Geometry check sheet. Reference: the model listing, model coordinates, mm. A direction names the side the tool comes from. Coordinates: 2 decimals unless noted, no trailing zeros. Write each loop counter-clockwise with the first axis right and the second up, starting at its lowest first coordinate (ties: lowest second). Pieces come first, ordered by that corner, then holes. Notation, with made-up numbers: (74.25, -0.75) -> (130.25, -0.75) arc R19 ccw to (130.25, 15.25) -> close; hole circle Ø2 at (-2, -17). An arc over 180 degrees is marked (long way). Use a Markdown table: item, result.
```python
from build123d import *

# Parameters (mm, degrees)
F1_DEPTH = 6.35
F2_R     = 6.35
F3_DEPTH = 6.35
F4_R     = 7.9375
F4_R_2   = 6.35
F5_DEPTH = 1.5875


with BuildPart() as f1:
    # F0 (on Front) → F1 (new body)
    with BuildSketch(Plane.XZ):
        with BuildLine():
            Line((-1.190625, 4.953), (-1.190625, 6.108039))
            ThreePointArc((-1.190625, 6.108039), (-2.381439, 5.749302), (-3.477137, 5.160935))
            Line((-3.477137, 5.160935), (-2.660401, 4.344199))
            Line((-2.660401, 4.344199), (-4.344199, 2.660401))
            Line((-4.344199, 2.660401), (-5.160935, 3.477137))
            ThreePointArc((-5.160935, 3.477137), (-5.749302, 2.381439), (-6.108039, 1.190625))
            Line((-6.108039, 1.190625), (-4.953, 1.190625))
            Line((-4.953, 1.190625), (-4.953, -1.190625))
            Line((-4.953, -1.190625), (-6.108039, -1.190625))
            ThreePointArc((-6.108039, -1.190625), (-5.749302, -2.381439), (-5.160935, -3.477137))
            Line((-5.160935, -3.477137), (-4.344199, -2.660401))
            Line((-4.344199, -2.660401), (-2.660401, -4.344199))
            Line((-2.660401, -4.344199), (-3.477137, -5.160935))
            ThreePointArc((-3.477137, -5.160935), (-2.381439, -5.749302), (-1.190625, -6.108039))
            Line((-1.190625, -6.108039), (-1.190625, -4.953))
            Line((-1.190625, -4.953), (1.190625, -4.953))
            Line((1.190625, -4.953), (1.190625, -6.108039))
            ThreePointArc((1.190625, -6.108039), (2.381439, -5.749302), (3.477137, -5.160935))
            Line((3.477137, -5.160935), (2.660401, -4.344199))
            Line((2.660401, -4.344199), (4.344199, -2.660401))
            Line((4.344199, -2.660401), (5.160935, -3.477137))
            ThreePointArc((5.160935, -3.477137), (5.749302, -2.381439), (6.108039, -1.190625))
            Line((6.108039, -1.190625), (4.953, -1.190625))
            Line((4.953, -1.190625), (4.953, 1.190625))
            Line((4.953, 1.190625), (6.108039, 1.190625))
            ThreePointArc((6.108039, 1.190625), (5.749302, 2.381439), (5.160935, 3.477137))
            Line((5.160935, 3.477137), (4.344199, 2.660401))
            Line((4.344199, 2.660401), (2.660401, 4.344199))
            Line((2.660401, 4.344199), (3.477137, 5.160935))
            ThreePointArc((3.477137, 5.160935), (2.381439, 5.749302), (1.190625, 6.108039))
            Line((1.190625, 6.108039), (1.190625, 4.953))
            Line((1.190625, 4.953), (-1.190625, 4.953))
        make_face()
    extrude(amount=F1_DEPTH)

    # F2 (on face) → F3 (join)
    with BuildSketch(Plane.XZ.offset(6.35)):
        Circle(F2_R)
        with BuildLine():
            Line((-3.477137, -5.160935), (-2.660401, -4.344199))
            Line((-2.660401, -4.344199), (-4.344199, -2.660401))
            Line((-4.344199, -2.660401), (-5.160935, -3.477137))
            ThreePointArc((-5.160935, -3.477137), (-5.749302, -2.381439), (-6.108039, -1.190625))
            Line((-6.108039, -1.190625), (-4.953, -1.190625))
            Line((-4.953, -1.190625), (-4.953, 1.190625))
            Line((-4.953, 1.190625), (-6.108039, 1.190625))
            ThreePointArc((-6.108039, 1.190625), (-5.749302, 2.381439), (-5.160935, 3.477137))
            Line((-5.160935, 3.477137), (-4.344199, 2.660401))
            Line((-4.344199, 2.660401), (-2.660401, 4.344199))
            Line((-2.660401, 4.344199), (-3.477137, 5.160935))
            ThreePointArc((-3.477137, 5.160935), (-2.381439, 5.749302), (-1.190625, 6.108039))
            Line((-1.190625, 6.108039), (-1.190625, 4.953))
            Line((-1.190625, 4.953), (1.190625, 4.953))
            Line((1.190625, 4.953), (1.190625, 6.108039))
            ThreePointArc((1.190625, 6.108039), (2.381439, 5.749302), (3.477137, 5.160935))
            Line((3.477137, 5.160935), (2.660401, 4.344199))
            Line((2.660401, 4.344199), (4.344199, 2.660401))
            Line((4.344199, 2.660401), (5.160935, 3.477137))
            ThreePointArc((5.160935, 3.477137), (5.749302, 2.381439), (6.108039, 1.190625))
            Line((6.108039, 1.190625), (4.953, 1.190625))
            Line((4.953, 1.190625), (4.953, -1.190625))
            Line((4.953, -1.190625), (6.108039, -1.190625))
            ThreePointArc((6.108039, -1.190625), (5.749302, -2.381439), (5.160935, -3.477137))
            Line((5.160935, -3.477137), (4.344199, -2.660401))
            Line((4.344199, -2.660401), (2.660401, -4.344199))
            Line((2.660401, -4.344199), (3.477137, -5.160935))
            ThreePointArc((3.477137, -5.160935), (2.381439, -5.749302), (1.190625, -6.108039))
            Line((1.190625, -6.108039), (1.190625, -4.953))
            Line((1.190625, -4.953), (-1.190625, -4.953))
            Line((-1.190625, -4.953), (-1.190625, -6.108039))
            ThreePointArc((-1.190625, -6.108039), (-2.381439, -5.749302), (-3.477137, -5.160935))
        make_face(mode=Mode.SUBTRACT)
        with BuildLine():
            Line((-4.344199, -2.660401), (-2.660401, -4.344199))
            Line((-2.660401, -4.344199), (-3.477137, -5.160935))
            ThreePointArc((-3.477137, -5.160935), (-2.381439, -5.749302), (-1.190625, -6.108039))
            Line((-1.190625, -6.108039), (-1.190625, -4.953))
            Line((-1.190625, -4.953), (1.190625, -4.953))
            Line((1.190625, -4.953), (1.190625, -6.108039))
            ThreePointArc((1.190625, -6.108039), (2.381439, -5.749302), (3.477137, -5.160935))
            Line((3.477137, -5.160935), (2.660401, -4.344199))
            Line((2.660401, -4.344199), (4.344199, -2.660401))
            Line((4.344199, -2.660401), (5.160935, -3.477137))
            ThreePointArc((5.160935, -3.477137), (5.749302, -2.381439), (6.108039, -1.190625))
            Line((6.108039, -1.190625), (4.953, -1.190625))
            Line((4.953, -1.190625), (4.953, 1.190625))
            Line((4.953, 1.190625), (6.108039, 1.190625))
            ThreePointArc((6.108039, 1.190625), (5.749302, 2.381439), (5.160935, 3.477137))
            Line((5.160935, 3.477137), (4.344199, 2.660401))
            Line((4.344199, 2.660401), (2.660401, 4.344199))
            Line((2.660401, 4.344199), (3.477137, 5.160935))
            ThreePointArc((3.477137, 5.160935), (2.381439, 5.749302), (1.190625, 6.108039))
            Line((1.190625, 6.108039), (1.190625, 4.953))
            Line((1.190625, 4.953), (-1.190625, 4.953))
            Line((-1.190625, 4.953), (-1.190625, 6.108039))
            ThreePointArc((-1.190625, 6.108039), (-2.381439, 5.749302), (-3.477137, 5.160935))
            Line((-3.477137, 5.160935), (-2.660401, 4.344199))
            Line((-2.660401, 4.344199), (-4.344199, 2.660401))
            Line((-4.344199, 2.660401), (-5.160935, 3.477137))
            ThreePointArc((-5.160935, 3.477137), (-5.749302, 2.381439), (-6.108039, 1.190625))
            Line((-6.108039, 1.190625), (-4.953, 1.190625))
            Line((-4.953, 1.190625), (-4.953, -1.190625))
            Line((-4.953, -1.190625), (-6.108039, -1.190625))
            ThreePointArc((-6.108039, -1.190625), (-5.749302, -2.381439), (-5.160935, -3.477137))
            Line((-5.160935, -3.477137), (-4.344199, -2.660401))
        make_face()
    extrude(amount=F3_DEPTH)

    # F4 (on face) → F5 (join)
    with BuildSketch(Plane.XZ.offset(12.7)):
        Circle(F4_R)
        Circle(F4_R_2, mode=Mode.SUBTRACT)
        Circle(F4_R_2)
    extrude(amount=F5_DEPTH)


solid = f1.part
```
Item 1: Section check B-B on z = -3.25. Record the boundary of the cut face in (x, y), then the cut area to 3 significant figures.
Answer block:
| item | result |
|---|---|
| outline | (-7.24, -14.29) -> (7.24, -14.29) -> (7.24, -12.7) -> (5.46, -12.7) -> (5.46, -6.35) -> (5.31, -6.35) -> (5.31, 0) -> (4.93, 0) -> (4.93, -6.35) -> (3.75, -6.35) -> (3.75, 0) -> (-3.75, 0) -> (-3.75, -6.35) -> (-4.93, -6.35) -> (-4.93, 0) -> (-5.31, 0) -> (-5.31, -6.35) -> (-5.46, -6.35) -> (-5.46, -12.7) -> (-7.24, -12.7) -> close |
| area | 145 mm^2 |
Item 2: Thickness scan on L1, parallel to Y at x = 0.25, z = 7.25; L2, parallel to Z at x = -0.25, y = -8; L3, parallel to Y at x = -4.75, z = 3.5. Record the ranges inside material, lowest first. Write a range as [from, to].
Answer block:
| item | result |
|---|---|
| L1 | y = [-14.29, -12.7] |
| L2 | z = [-6.35, 6.35] |
| L3 | y = [-14.29, -6.35] |
Item 3: Section check A-A on x = 0. Record the boundary of the cut face in (y, z).
Answer block:
| item | result |
|---|---|
| outline | (-14.29, -7.94) -> (-12.7, -7.94) -> (-12.7, -6.35) -> (-6.35, -6.35) -> (-6.35, -4.95) -> (0, -4.95) -> (0, 4.95) -> (-6.35, 4.95) -> (-6.35, 6.35) -> (-12.7, 6.35) -> (-12.7, 7.94) -> (-14.29, 7.94) -> close |
Item 4: Mould release check, pull along X, two halves, no side actions. Record for faces 1 (the flat face through (5.5, -3.1, -1.191)), 2 (the flat face through (-3.074, -3.131, 4.758)), 3 (the flat face through (-1.191, -3.1, 5.5)), 4 (the flat face through (3.514, -3.131, 3.491)): +X half, -X half, draft (parallel to the pull), parting line (faces both ways), or undercut.
Answer block:
| item | result |
|---|---|
| face 1 | draft |
| face 2 | -X half |
| face 3 | undercut |
| face 4 | undercut |
Item 5: Section check D-D on z = 0. Record the boundary of the cut face in (x, y).
Answer block:
| item | result |
|---|---|
| outline | (-7.94, -14.29) -> (7.94, -14.29) -> (7.94, -12.7) -> (6.35, -12.7) -> (6.35, -6.35) -> (4.95, -6.35) -> (4.95, 0) -> (-4.95, 0) -> (-4.95, -6.35) -> (-6.35, -6.35) -> (-6.35, -12.7) -> (-7.94, -12.7) -> close |
Item 6: Depth check by flat-ended pin: P1, Ø0.6, axis at y = -2, z = -5.5, coming from the -X side; P2, Ø0.7, axis at x = 0, y = -3.5, coming from the -Z side; P3, Ø5, axis at x = 6, y = -5.5, coming from the +Z side. Enter the tip coordinate at first touch or a pass-through.
Answer block:
| item | result |
|---|---|
| P1 | stops at x = -3.42 |
| P2 | stops at z = -4.95 |
| P3 | stops at z = 5.2 |
Item 7: Section check C-C on y = -9. Record the boundary of the cut face in (x, z).
Answer block:
| item | result |
|---|---|
| outline | circle Ø12.7 at (0, 0) |
Item 8: Tool access check on faces 5 (the flat face through (3.074, -3.131, -4.758)), 6 (the flat face through (-4.953, -3, 0)), 7 (the cylindrical face through (-2.365, -3.131, 5.756)). Record the directions out of +Z, -Z, +X, -X, +Y, -Y that give a thin tool (end or side, any length) a straight path to the whole face; none if there is none.
Answer block:
| item | result |
|---|---|
| face 5 | +X, +Y |
| face 6 | -X, +Y |
| face 7 | +Z, -X, +Y |
